from build123d import *

# Parameters (mm, degrees)
F1_DEPTH = 69.07994
F2_R     = 2
F3_R     = 2


with BuildPart() as f1:
    # F0 (on Front) → F1 (new body)
    with BuildSketch(Plane.XZ):
        with BuildLine():
            Line((0, -2), (0, 0))
            ThreePointArc((0, 0), (-19.035896, 6.244577), (-38.958142, 8.357436))
            Line((-38.958142, 8.357436), (-40.958142, 8.357436))
            Line((-40.958142, 8.357436), (-44, 0))
            Line((-44, 0), (-46, 0))
            Line((-46, 0), (-44.180149, 5))
            Line((-44.180149, 5), (-46.180149, 5))
            Line((-46.180149, 5), (-48, 0))
            Line((-48, 0), (-58, 0))
            Line((-58, 0), (-58, 5))
            Line((-58, 5), (-60, 5))
            Line((-60, 5), (-60, -2))
            Line((-60, -2), (0, -2))
        make_face()
    extrude(amount=-F1_DEPTH)

    # F2
    f2_edges = [f1.edges().sort_by_distance(p)[0] for p in [
        (-48, 34.53997, 0),
    ]]
    fillet(f2_edges, radius=F2_R)

    # F3
    f3_edges = [f1.edges().sort_by_distance(p)[0] for p in [
        (-58, 34.53997, 0),
    ]]
    fillet(f3_edges, radius=F3_R)


solid = f1.part
Geometry check sheet. Reference: the model listing, model coordinates, mm. A direction names the side the tool comes from. Round coordinates to 2 decimals unless told otherwise and drop trailing zeros. Order: outer loops, then holes, each group sorted by start corner. A loop starts at its lowest first (then second) coordinate and runs counter-clockwise, first axis right, second up. Notation, with made-up numbers: M 77.5,85.25 L 85.5,85.25 A28 cw 85.5,122.25 Z; hole C 64,77 d3. An arc over 180 degrees is marked long. Write each question's results on one line, items separated by ' | '. Start each with the question number.
1. Cross-section at A-A on z = 3.5. Record the boundary of the cut face in (x, y).
2. Cross-section at B-B on y = 62.5. Record the boundary of the cut face in (x, z).
3. Go/stop test with flat-tipped pins: P1, Ø0.6, axis at x = -45, y = 51.5, coming from the +Z side; P2, Ø3.5, axis at y = 49, z = 3, coming from the +X side; P3, Ø8, axis at x = -19, y = 22.5, coming from the +Z side. Record where each tip stops, or that it passes through.
4. Draft check along X on faces 1 (the face through (-59, 34, 5)), 2 (the face through (-18.761, 34.056, 6.185)), 3 (the face through (-57.4, 35.02, 0.57)). Enter one of: pulls with the +X half, pulls with the -X half, needs draft (parallel to the pull), parting line crosses it, or undercut.
5. Cross-section at C-C on x = -51. Record the boundary of the cut face in (y, z), plus the area to 3 significant figures.
6. Set-up check for faces 4 (the face through (-45, 34, 5)), 5 (the face through (-53, 34, 0)), 6 (the face through (-45.1, 34.06, 2.47)): record each of +Z, -Z, +X, -X, +Y, -Y from which the full face is reachable in a straight line by a thin tool's end or side.
7. Material ranges on L1, parallel to X at y = 34, z = 0.5; L2, parallel to X at y = 25, z = 0.25; L3, parallel to Z at x = -55, y = 4.5, recorded low to high. Write a range as from..to.
Resolved:
1) outline: M -60,0 L -58,0 L -58,69.08 L -60,69.08 Z; M -46.73,0 L -44.73,0 L -44.73,69.08 L -46.73,69.08 Z; M -42.73,0 L -8.97,0 L -8.97,69.08 L -42.73,69.08 Z
2) outline: M -60,-2 L 0,-2 L 0,0 A94.98 ccw -38.96,8.36 L -40.96,8.36 L -44,0 L -46,0 L -44.18,5 L -46.18,5 L -47.52,1.32 A2 cw -49.4,0 L -56,0 A2 cw -58,2 L -58,5 L -60,5 Z
3) P1: z = 5 | P2: x = -2.91 | P3: z = 7.01
4) face 1: needs draft | face 2: pulls with the +X half | face 3: undercut
5) outline: M 0,-2 L 69.08,-2 L 69.08,0 L 0,0 Z | area: 138 mm2
6) face 4: +Z, -X, +Y, -Y | face 5: +Z, +Y, -Y | face 6: +Y, -Y
7) L1: -60..-57.32, -48.08..-45.82, -43.82..-1.13 | L2: -60..-56.97, -48.43..-45.91, -43.91..-0.56 | L3: -2..0
